Verification items for the finished model (mm, model axes). Face numbers are marked on the shaded views. Round coordinates to 2 decimals unless told otherwise and drop trailing zeros. Write each loop counter-clockwise with the first axis right and the second up, starting at its lowest first coordinate (ties: lowest second). Pieces come first, ordered by that corner, then holes. Notation, with made-up numbers: (44, 56) - (81, 56) arc R23 cw to (81, 81) - close; hole circle Ø10 at (12, 55.25). An arc over 180 degrees is marked (long way). Answer as a JSON object with one key per item and string values. Group by question number.
1) Mould release check, pull along Y, two halves, no side actions. Record for the marked faces 1, 2, 3 and 4: +Y half, -Y half, draft (parallel to the pull), parting line (faces both ways), or undercut.
2) Section check B-B (y = -5.5). Enter the section's corners in (x, z), then the cut area to 3 significant figures.
3) Thickness scan on line 1 (Y direction, x = 18.25, z = 0.25); line 2 (Y direction, x = 18.75, z = 1.65); line 3 (X direction, y = -28, z = 1.6). Record the ranges inside material, lowest first.
4) Go/stop test with flat-tipped pins: pin 1 Ø1 at (y, z) = (-14, 1) entering from +X; pin 2 Ø1.1 at (y, z) = (3.5, 0.5) entering from -X; pin 3 Ø0.8 at (y, z) = (3.5, 0.5) entering from +X. Record where each tip stops, or that it passes through.
5) Section check A-A (z = 2.35). State how many separate pieces and enclosed holes the cut face has, then the cut area to 3 significant figures.
6) Section check C-C (x = 15). Enter the section's corners in (y, z).
```python
from build123d import *

# Parameters (mm, degrees)
SKETCH_1_R          = 1.35
SKETCH_1_R_2        = 1.65
SKETCH_1_R_3        = 1.3
EXTRUDE_1_DEPTH     = 3
SKETCH_2_R          = 1.65
CUT_EXTRUDE_1_DEPTH = 40.58429055
CUT_EXTRUDE_2_DEPTH = 1


with BuildPart() as part:
    # 草图1 → 凸台-拉伸1 (new body)
    with BuildSketch(Plane(origin=(0, 0, 0), x_dir=(-1, 0, 0), z_dir=(0, 0, -1))):
        with BuildLine():
            Line((3.311115848, 16.021732214), (3.313115848, 16.021732214))
            ThreePointArc((3.313115848, 16.021732214), (1.422584465, 20.809546819), (-3.619383376, 19.772320768))
            ThreePointArc((-3.619383376, 19.772320768), (-3.907451025, 19.356483629), (-4.140741668, 18.907619539))
            ThreePointArc((-4.140741668, 18.907619539), (-9.493299368, 12.888445888), (-17.351741668, 11.120619539))
            ThreePointArc((-17.351741668, 11.120619539), (-19.703460244, 10.604408599), (-21.333741668, 8.832619539))
            ThreePointArc((-21.333741668, 8.832619539), (-21.651545732, 6.446374123), (-20.542741668, 4.309619539))
            ThreePointArc((-20.542741668, 4.309619539), (-9.614805592, -11.161234041), (-4.459741668, -29.387380461))
            ThreePointArc((-4.459741668, -29.387380461), (-3.626617209, -31.434284825), (-1.833741668, -32.726380461))
            ThreePointArc((-1.833741668, -32.726380461), (0.370527809, -32.871130249), (2.315258332, -31.823380461))
            ThreePointArc((2.315258332, -31.823380461), (3.407459975, -29.901725556), (3.313258332, -27.693380461))
            ThreePointArc((3.313258332, -27.693380461), (-0.247316641, -5.861423686), (3.295002421, 15.973502613))
            Line((3.295002421, 15.973502613), (3.311115848, 16.021732214))
        make_face()
        with Locations(Location((-17.711384152, 7.136232214, 0), (0, 0, 180))):
            Circle(SKETCH_1_R, mode=Mode.SUBTRACT)
        with Locations(Location((-0.480884152, -28.962767786, 0), (0, 0, 180))):
            Circle(SKETCH_1_R_2, mode=Mode.SUBTRACT)
        with Locations(Location((-0.480884152, 17.291232214, 0), (0, 0, 180))):
            Circle(SKETCH_1_R_3, mode=Mode.SUBTRACT)
    extrude(amount=-EXTRUDE_1_DEPTH)

    # 草图2 → 切除-拉伸1 (cut, through all)
    with BuildSketch(Plane.XY.offset(3)):
        with Locations((0.480884152, 17.291232214)):
            Circle(SKETCH_2_R)
        with Locations((17.711384152, 7.136232214)):
            Circle(SKETCH_2_R)
    extrude(amount=-CUT_EXTRUDE_1_DEPTH, mode=Mode.SUBTRACT)

    # 草图3 → 切除-拉伸2 (cut)
    # profile 1 of 2: a face of its own
    with BuildSketch(Plane(origin=(0, 0, 0), x_dir=(-1, 0, 0), z_dir=(0, 0, -1))):
        Polygon((-9.088408768, 5.724720745), (-8.441273352, 5.724720745), (-8.441273352, 2.224720745), (-8.755375916, 2.224720745), (-8.755375916, 5.365746386), (-9.293837454, 5.365746386), align=None)
    # profile 2 of 2: a face of its own
    with BuildSketch(Plane(origin=(0, 0, 0), x_dir=(-1, 0, 0), z_dir=(0, 0, -1))):
        with BuildLine():
            add(Edge.make_bspline(
                [(-7.1399913, 3.973318501), (-7.139663282, 4.029415889), (-7.139026102, 4.138385873), (-7.131937681, 4.297170516), (-7.120162339, 4.446130805), (-7.104024966, 4.585273871), (-7.084386986, 4.714635635), (-7.058171499, 4.833870392), (-7.028358697, 4.943529999), (-6.993806251, 5.043972047), (-6.954818462, 5.13654975), (-6.912384201, 5.222974952), (-6.864819407, 5.303116884), (-6.814842494, 5.378254674), (-6.760430422, 5.447158369), (-6.703131632, 5.510801032), (-6.640709755, 5.567711782), (-6.575286747, 5.619558085), (-6.506270283, 5.665007556), (-6.435627617, 5.705040295), (-6.362872511, 5.739240162), (-6.287806328, 5.766130598), (-6.21110377, 5.788341445), (-6.132496703, 5.803530392), (-6.051855339, 5.813087301), (-5.997423905, 5.814000969), (-5.969819025, 5.814464335)],
                knots=[0, 0, 0, 0, 1.646270934, 3.197905019, 4.663502075, 6.030701355, 7.308322542, 8.50163776, 9.611534131, 10.641858119, 11.616356847, 12.558055219, 13.465016945, 14.349605745, 15.204443733, 16.039544428, 16.859896111, 17.680448484, 18.487036065, 19.28249412, 20.06191084, 20.843045899, 21.620316918, 22.403196591, 23.190181807, 24, 24, 24, 24], degree=3))
            add(Edge.make_bspline(
                [(-5.969819025, 5.814464335), (-5.941983546, 5.81397652), (-5.886627537, 5.813006409), (-5.804787162, 5.803682466), (-5.72483748, 5.788211343), (-5.647119342, 5.766290368), (-5.570994355, 5.739094692), (-5.497057948, 5.705007575), (-5.424850866, 5.665328707), (-5.355520578, 5.61870483), (-5.288305963, 5.566722554), (-5.224858, 5.507959885), (-5.165170914, 5.443010166), (-5.108495609, 5.372568302), (-5.056440012, 5.295283217), (-5.006866579, 5.212499107), (-4.962494544, 5.122768242), (-4.919759868, 5.027587775), (-4.882872882, 4.924324116), (-4.849606636, 4.813559355), (-4.822727668, 4.693985168), (-4.800338395, 4.566228923), (-4.782993499, 4.42982144), (-4.770360857, 4.285055124), (-4.763687772, 4.131834734), (-4.762431071, 4.027076885), (-4.761786172, 3.973318501)],
                knots=[0, 0, 0, 0, 0.810914788, 1.612654377, 2.396697861, 3.181598691, 3.963628158, 4.749916497, 5.551656086, 6.361998678, 7.18212741, 8.025565596, 8.878627764, 9.750805457, 10.657531673, 11.591944965, 12.560506719, 13.57287815, 14.630710178, 15.753379473, 16.941251878, 18.199788006, 19.531962791, 20.947069417, 22.433333509, 24, 24, 24, 24], degree=3))
            add(Edge.make_bspline(
                [(-4.761786172, 3.973318501), (-4.762437757, 3.919794594), (-4.763707343, 3.815505442), (-4.770286049, 3.662974466), (-4.783244681, 3.518976423), (-4.799454669, 3.383165961), (-4.821905632, 3.256108342), (-4.849510798, 3.137363893), (-4.880161121, 3.026419822), (-4.917995915, 2.92418501), (-4.959406625, 2.829233287), (-5.004461822, 2.740566139), (-5.052731648, 2.657399846), (-5.105320393, 2.580400099), (-5.161373806, 2.509021442), (-5.222091595, 2.444523819), (-5.28576218, 2.385353148), (-5.353174596, 2.33270152), (-5.423586147, 2.286616715), (-5.495545224, 2.245402865), (-5.570328607, 2.21217017), (-5.64624156, 2.183635129), (-5.724369926, 2.161834677), (-5.804616317, 2.146760822), (-5.886572553, 2.136188973), (-5.941974118, 2.135382493), (-5.969819025, 2.134977155)],
                knots=[0, 0, 0, 0, 1.561518951, 3.042555995, 4.452378317, 5.7783523, 7.031515105, 8.214008947, 9.334062868, 10.386615937, 11.391082383, 12.354592575, 13.286541444, 14.194233754, 15.072674879, 15.931287219, 16.775624067, 17.606195743, 18.42308326, 19.229000347, 20.022332153, 20.807536673, 21.593273796, 22.3848459, 23.188221202, 24, 24, 24, 24], degree=3))
            add(Edge.make_bspline(
                [(-5.969819025, 2.134977155), (-5.997423139, 2.135443511), (-6.051853064, 2.136363073), (-6.132505489, 2.145876804), (-6.210787932, 2.161172307), (-6.287086686, 2.182588911), (-6.361793202, 2.208803748), (-6.433889488, 2.242957431), (-6.504177172, 2.2822915), (-6.572468728, 2.327086922), (-6.637480889, 2.378408605), (-6.699579494, 2.435172894), (-6.757204513, 2.498796305), (-6.810838609, 2.568274228), (-6.861812697, 2.64296747), (-6.90870207, 2.723895843), (-6.952072925, 2.810738454), (-6.991716415, 2.904056365), (-7.026865079, 3.005211292), (-7.057912787, 3.115360471), (-7.082426944, 3.235476107), (-7.1034099, 3.364593474), (-7.120334283, 3.503267405), (-7.131888608, 3.651573183), (-7.139029923, 3.809418392), (-7.139664993, 3.917688166), (-7.1399913, 3.973318501)],
                knots=[0, 0, 0, 0, 0.810891512, 1.598919785, 2.382837074, 3.152667961, 3.926044502, 4.706494248, 5.493654104, 6.291793342, 7.103789334, 7.925228297, 8.761435821, 9.622817696, 10.50288917, 11.416980706, 12.369136599, 13.353924996, 14.394355917, 15.514179734, 16.714354668, 17.994756427, 19.357759367, 20.818452758, 22.365282078, 24, 24, 24, 24], degree=3))
        make_face()
        with BuildLine():
            add(Edge.make_bspline(
                [(-6.825888736, 3.974720745), (-6.825769289, 3.927972046), (-6.825537466, 3.837242001), (-6.819481265, 3.70539874), (-6.811231033, 3.582428412), (-6.800589736, 3.468174875), (-6.784786788, 3.363024863), (-6.76708, 3.26625518), (-6.74553191, 3.178377942), (-6.720036892, 3.098790132), (-6.690997795, 3.026141063), (-6.659291932, 2.958539848), (-6.625231209, 2.895187912), (-6.587112058, 2.836654303), (-6.545596995, 2.782748139), (-6.501623736, 2.732515307), (-6.453551152, 2.687718326), (-6.387047409, 2.633991471), (-6.299250935, 2.578472337), (-6.18863048, 2.530126247), (-6.074962029, 2.499743791), (-5.997810778, 2.495880035), (-5.959302198, 2.493951514)],
                knots=[0, 0, 0, 0, 1.459021318, 2.831673884, 4.118529203, 5.306027144, 6.411944654, 7.436330062, 8.375795394, 9.233974572, 10.042671642, 10.816086306, 11.563610507, 12.285937304, 12.993564865, 13.685989202, 14.367179055, 15.041617293, 16.353048772, 17.594441528, 18.799311195, 20, 20, 20, 20], degree=3))
            add(Edge.make_bspline(
                [(-5.959302198, 2.493951514), (-5.920544526, 2.495549295), (-5.843109203, 2.498741558), (-5.729975408, 2.529540295), (-5.620145138, 2.576009835), (-5.534073197, 2.63095734), (-5.468590654, 2.68328567), (-5.421673664, 2.727900318), (-5.378611615, 2.777856185), (-5.337769541, 2.831755481), (-5.300310465, 2.890627965), (-5.266247327, 2.954190541), (-5.23516398, 3.022619718), (-5.217454934, 3.070389458), (-5.208400756, 3.094812892)],
                knots=[0, 0, 0, 0, 1.353760809, 2.704726607, 4.075137775, 5.516104923, 6.260822281, 7.007110065, 7.778089737, 8.566572457, 9.372053459, 10.217411131, 11.088608312, 12, 12, 12, 12], degree=3))
            add(Edge.make_bspline(
                [(-5.208400756, 3.094812892), (-5.197848988, 3.126042632), (-5.176424374, 3.189452396), (-5.1488126, 3.287816048), (-5.1270672, 3.391018812), (-5.107503835, 3.498443929), (-5.094150779, 3.61088363), (-5.083402966, 3.727990014), (-5.077072279, 3.849851376), (-5.076287527, 3.932646367), (-5.075888736, 3.974720745)],
                knots=[0, 0, 0, 0, 0.884706709, 1.796334032, 2.740027952, 3.714592787, 4.726048262, 5.777819803, 6.87074269, 8, 8, 8, 8], degree=3))
            add(Edge.make_bspline(
                [(-5.075888736, 3.974720745), (-5.076438926, 4.016788318), (-5.077515213, 4.099081482), (-5.081629201, 4.219599663), (-5.092252775, 4.334067424), (-5.104051894, 4.442977897), (-5.121449115, 4.545728199), (-5.140206922, 4.643178505), (-5.165408135, 4.734121529), (-5.19232791, 4.819981111), (-5.223138305, 4.899781766), (-5.257054039, 4.973895552), (-5.293275798, 5.042680277), (-5.332618039, 5.105947218), (-5.374613722, 5.163979761), (-5.420371271, 5.215614356), (-5.468075644, 5.262451324), (-5.53489283, 5.315913893), (-5.622367119, 5.370425588), (-5.731212767, 5.420591348), (-5.844483411, 5.449399641), (-5.921056865, 5.453461328), (-5.959302198, 5.455489976)],
                knots=[0, 0, 0, 0, 1.31362396, 2.569729283, 3.763502607, 4.902122613, 5.988968491, 7.01645872, 7.998833611, 8.933434873, 9.825090667, 10.667526885, 11.477055099, 12.250526234, 12.991942729, 13.710640831, 14.402115721, 15.076753259, 16.378508321, 17.609869233, 18.806226677, 20, 20, 20, 20], degree=3))
            add(Edge.make_bspline(
                [(-5.959302198, 5.455489976), (-5.99801279, 5.453458529), (-6.075504496, 5.449391935), (-6.18995245, 5.420698681), (-6.299656802, 5.370685716), (-6.386899777, 5.315733343), (-6.453763563, 5.263395032), (-6.500846256, 5.218008578), (-6.544992429, 5.168362323), (-6.585660129, 5.113960408), (-6.623749412, 5.055495041), (-6.658730425, 4.992506276), (-6.690247754, 4.924674912), (-6.71933229, 4.852058477), (-6.744905078, 4.772477532), (-6.765999042, 4.684708539), (-6.785486095, 4.588246647), (-6.799281364, 4.482527139), (-6.811545119, 4.368244986), (-6.819426467, 4.244967667), (-6.825557725, 4.112903287), (-6.825776189, 4.021704128), (-6.825888736, 3.974720745)],
                knots=[0, 0, 0, 0, 1.207732386, 2.417664972, 3.655092373, 4.956220595, 5.625982001, 6.301752483, 6.994047911, 7.697131622, 8.419323945, 9.170223765, 9.943494443, 10.752040957, 11.610060368, 12.549350801, 13.567764191, 14.679664412, 15.874934091, 17.154273443, 18.533957287, 20, 20, 20, 20], degree=3))
        make_face(mode=Mode.SUBTRACT)
    extrude(amount=-CUT_EXTRUDE_2_DEPTH, mode=Mode.SUBTRACT)


solid = part.part
```
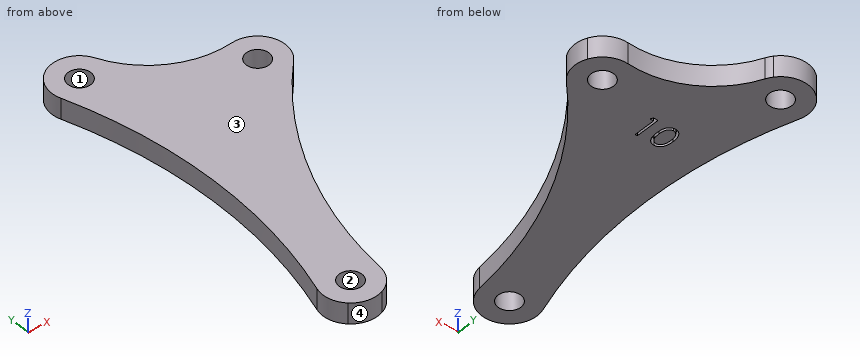
Returned:
{
 "1": {"face 1": "undercut", "face 2": "undercut", "face 3": "draft", "face 4": "-Y half"},
 "2": {"outline": "(0.25, 0) - (12.73, 0) - (12.73, 3) - (0.25, 3) - close", "area": "37.4 mm2"},
 "3": {"line 1": "1.87 to 5.58, 8.7 to 11.1", "line 2": "2.43 to 5.85, 8.42 to 11", "line 3": "-3.4 to -0.86, 1.82 to 4.62"},
 "4": {"pin 1": "x = 8.56", "pin 2": "x = -0.47", "pin 3": "x = 20.14"},
 "5": {"separate pieces": "1", "enclosed holes": "3", "area": "608 mm2"},
 "6": {"outline": "(-2.16, 0) - (11.12, 0) - (11.12, 3) - (-2.16, 3) - close"}
}
